Input: part model. Units: mm. Frame: model coordinates. A direction names the side the tool comes from. Round coordinates to 2 decimals unless told otherwise and drop trailing zeros. Loops run counter-clockwise (first coordinate to the right, second up) from the corner with the lowest first, then second, coordinate; pieces in that order, holes last. Notation, with made-up numbers: M -4,55.25 L 4,55.25 A13 cw 4,74.25 Z; hole C -4,-5.75 d2. An arc over 180 degrees is marked long. Use one line per item in the form item = value. Start each with the question number.
Q1. Section query C-C, the plane z = 1.1. State how many separate pieces and enclosed holes the cut face has, and give its area (3 significant figures).
Q2. Ray query, line 1 along Y through (x, z) = (-352.5, 0.35); line 2 along Y through (x, z) = (-354.75, 0.7); line 3 along Y through (x, z) = (-354.5, 2.95). Return the intervals inside material, ascending.
Q3. Section query B-B, the plane y = 240. Output: boundary loops of the cut face in (x, z).
Q4. Mould query, pull axis Y, two halves, no side actions, for faces 1 (the flat face through (-357, 218.342, 1)), 2 (the flat face through (-346.824, 186.168, 1.479)), 3 (the flat face through (-356, 210, 0)), 4 (the flat face through (-357, 251.556, 1)). Classes: pulls with the +Y half, pulls with the -Y half, needs draft (parallel to the pull), parting line crosses it, or undercut.
Q5. First-contact query: P1, Ø1.5, axis at x = -356.55, y = 243.88, coming from the -Z side; P2, Ø1, axis at y = 230, z = 0.5, coming from the +X side; P3, Ø1.5, axis at y = 169.5, z = 2, coming from the -X side. Flat tips, straight axial feed; report the tip coordinate or a pass-through.
Q6. Section query A-A, the plane x = -353. Output: boundary loops of the cut face in (y, z).
Q7. Section query D-D, the plane x = -365. Output: boundary loops of the cut face in (y, z), and give its area (3 significant figures).
Q8. Access query for faces 5 (the flat face through (-363.785, 172, 1)), 6 (the flat face through (-362.501, 230, 1)), 7 (the flat face through (-357, 167.154, 1)). Directions: +Z, -Z, +X, -X, +Y, -Y. A direction counts if a zero-diameter tool reaches every point of the face in a straight line with its end or side. Return the directions, or none.
```python
from build123d import *

# Parameters (mm, degrees)
SKETCH1_R           = 0.85
SKETCH1_R_2         = 3
SKETCH1_W           = 11.7094
SKETCH1_H           = 23.7998
BOSS_EXTRUDE3_DEPTH = 3
SKETCH2_R           = 1.0009
CUT_EXTRUDE1_DEPTH  = 447.747926613


with BuildPart() as part:
    # Sketch1 → Boss-Extrude3 (new body)
    with BuildSketch(Plane.XY):
        Polygon((-363.784573438, 176.492478394), (-369.180567886, 195.576225703), (-369.180567886, 251.55599422), (-343.853730339, 251.55599422), (-343.806464443, 195.576225703), (-349.928026562, 176.492478394), (-349.928026562, 167.153932289), (-363.784573438, 167.153932289), align=None)
        with Locations((-356.653301567, 216.60430982)):
            Circle(SKETCH1_R, mode=Mode.SUBTRACT)
        with Locations((-356.547049339, 243.88030982)):
            Circle(SKETCH1_R, mode=Mode.SUBTRACT)
        with Locations((-356.8563, 181.55599422)):
            Circle(SKETCH1_R_2, mode=Mode.SUBTRACT)
        with Locations((-356.646530889, 230.24230982)):
            Rectangle(SKETCH1_W, SKETCH1_H, mode=Mode.SUBTRACT)
    extrude(amount=BOSS_EXTRUDE3_DEPTH)

    # Sketch2 → Cut-Extrude1 (cut, through all)
    with BuildSketch(Plane.XY.offset(3)):
        with Locations((-356.8563, 171.35599422)):
            Circle(SKETCH2_R)
        with Locations((-356.8563, 175.20599422)):
            Circle(SKETCH2_R)
        with Locations((-356.8563, 187.90599422)):
            Circle(SKETCH2_R)
        with Locations((-356.8563, 191.75599422)):
            Circle(SKETCH2_R)
    extrude(amount=-CUT_EXTRUDE1_DEPTH, mode=Mode.SUBTRACT)


solid = part.part
```
Results found:
q1.separate_pieces = 1
q1.enclosed_holes = 8
q1.area = 1,600 mm²
q2.line_1 = 167.15 to 218.34, 242.14 to 251.56
q2.line_2 = 167.15 to 179.42, 183.69 to 218.34, 242.14 to 251.56
q2.line_3 = 167.15 to 179.7, 183.41 to 218.34, 242.14 to 251.56
q3.outline = M -369.18,0 L -362.5,0 L -362.5,3 L -369.18,3 Z; M -350.79,0 L -343.84,0 L -343.84,3 L -350.79,3 Z
q4.face_1 = undercut
q4.face_2 = pulls with the -Y half
q4.face_3 = needs draft
q4.face_4 = pulls with the +Y half
q5.P1 = through
q5.P2 = -343.84
q5.P3 = -363.78
q6.outline = M 167.15,0 L 218.34,0 L 218.34,3 L 167.15,3 Z; M 242.14,0 L 251.56,0 L 251.56,3 L 242.14,3 Z
q7.outline = M 180.79,0 L 251.56,0 L 251.56,3 L 180.79,3 Z
q7.area = 212 mm²
q8.face_5 = +Z, -Z, -X, -Y
q8.face_6 = +Z, -Z
q8.face_7 = +Z, -Z, +X, -X, -Y
